For this review, take the finished solid that the model builds, in its own axes (mm). A direction names the side the tool comes from. Round coordinates to 2 decimals unless told otherwise and drop trailing zeros. Order: outer loops, then holes, each group sorted by start corner. A loop starts at its lowest first (then second) coordinate and runs counter-clockwise, first axis right, second up. Notation, with made-up numbers: (64.5, 67.25) - (79.5, 67.25) arc R16 ccw to (79.5, 85.25) - close; hole circle Ø9 at (68.5, -28). An arc over 180 degrees is marked (long way). One line per question, with ' | ' between items.
```python
from build123d import *

# Parameters (mm, degrees)
SKETCH_1_W      = 105
SKETCH_1_H      = 80
EXTRUDE_1_DEPTH = 1.702337868


with BuildPart() as part:
    # 草图1 → 凸台-拉伸1 (new body)
    with BuildSketch(Plane(origin=(0, 0, 0), x_dir=(1, 0, 0), z_dir=(0, 1, 0))):
        Rectangle(SKETCH_1_W, SKETCH_1_H)
        Polygon((38.759288178, 35), (37.759288178, 34), (36.759288178, 35), (37.759288178, 36), align=None, mode=Mode.SUBTRACT)
        Polygon((-37.759288178, 34), (-36.759288178, 35), (-37.759288178, 36), (-38.759288178, 35), align=None, mode=Mode.SUBTRACT)
        Polygon((37.759288178, -36), (38.759288178, -35), (37.759288178, -34), (36.759288178, -35), align=None, mode=Mode.SUBTRACT)
        Polygon((-38.759288178, -35), (-37.759288178, -34), (-36.759288178, -35), (-37.759288178, -36), align=None, mode=Mode.SUBTRACT)
        with BuildLine():
            Line((-7.5, -39), (7.5, -39))
            ThreePointArc((7.5, -39), (11.5, -35), (7.5, -31))
            Line((7.5, -31), (-7.5, -31))
            ThreePointArc((-7.5, -31), (-11.5, -35), (-7.5, -39))
        make_face(mode=Mode.SUBTRACT)
    extrude(amount=EXTRUDE_1_DEPTH)


solid = part.part
```
(1) Mouldability with a two-part tool opening along X and no side actions: class faces 1 (the flat face through (-1, 1.702, -1)), 2 (the cylindrical face through (-11.5, 0.8, 34.9)) as released by +X, released by -X, zero draft, split by the parting line, or undercut.
Output values:
face 1: zero draft | face 2: undercut
(2) For probe 1 along Z at (x, y) = (-5, 0.25); probe 2 along Z at (x, y) = (37, 0.7); probe 3 along Z at (x, y) = (10, 0.5), list the stretches that pass through material, from the lowest coordinate up. Write a range as [from, to].
Output values:
probe 1: [-40, 31], [39, 40] | probe 2: [-40, -35.24], [-34.76, 34.76], [35.24, 40] | probe 3: [-40, 31.88], [38.12, 40]
(3) For faces 3 (the flat face through (-1, 0, -1)), 4 (the cylindrical face through (11.5, 0.8, 35.1)), list the 3-axis set-ups (+Z, -Z, +X, -X, +Y, -Y) from which the entire face can be reached by the end or side of a thin tool; tool diameter is ignored.
Output values:
face 3: +Z, -Z, +X, -X, -Y | face 4: +Y, -Y
(4) We need section A-A on y = 0.75. State the section outline as (x, z) points.
Output values:
outline: (-52.5, -40) - (52.5, -40) - (52.5, 40) - (-52.5, 40) - close; hole (-38.76, -35) - (-37.76, -36) - (-36.76, -35) - (-37.76, -34) - close; hole (-38.76, 35) - (-37.76, 34) - (-36.76, 35) - (-37.76, 36) - close; hole (-7.5, 31) - (7.5, 31) arc R4 ccw to (7.5, 39) - (-7.5, 39) arc R4 ccw to start; hole (36.76, -35) - (37.76, -36) - (38.76, -35) - (37.76, -34) - close; hole (36.76, 35) - (37.76, 34) - (38.76, 35) - (37.76, 36) - close
